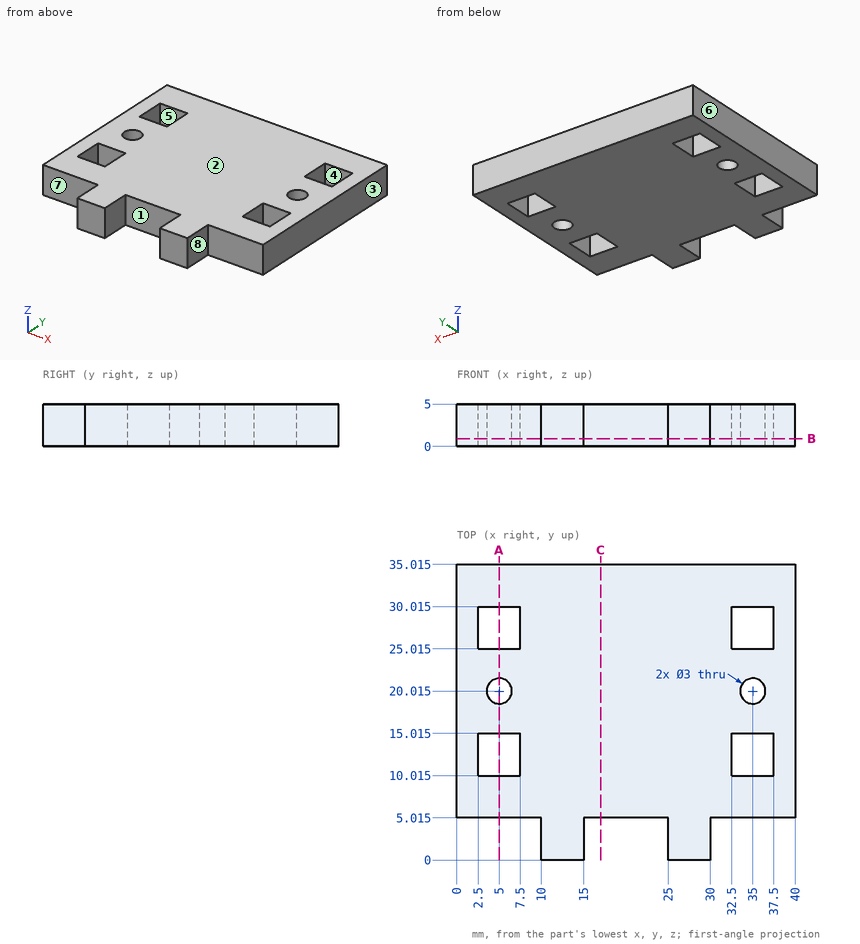
Part print with two shaded views. Sizes in mm from the minimum x, y, z corner. A direction names the side the tool comes from. Round coordinates to 2 decimals unless told otherwise and drop trailing zeros. Order: outer loops, then holes, each group sorted by start corner. A loop starts at its lowest first (then second) coordinate and runs counter-clockwise, first axis right, second up. Notation, with made-up numbers: M 62.5,62.25 L 112.5,62.25 A7 cw 112.5,71.25 Z; hole C -19,31 d9. An arc over 180 degrees is marked long. Use CSV: the item, a comma, the result in double quotes. Start each with the question number.
(1) Tool access for the marked faces 5, 6, 7 and 8: list every direction of +Z, -Z, +X, -X, +Y, -Y with a clear straight run to the whole face (end or side of a thin tool).
(2) Flat gauge pin, fed straight in: P1, Ø1.5, axis at x = 35, z = 3, coming from the -Y side (1 decimal). Where does the tip first touch, or does it go through?
(3) Cut at A-A on x = 5. List the corners of the cut face in (y, z) (1 decimal).
(4) Cut at C-C on x = 17. List the corners of the cut face in (y, z) (1 decimal), then the cut area to 3 significant figures.
(5) Cut at B-B on z = 0.9. State how many separate pieces and enclosed holes the cut face has, then the cut area to 3 significant figures.
(6) Drill centre lines: probe 1 along Y at (x, z) = (35, 2.4) (1 decimal); probe 2 along X at (y, z) = (13, 0.5); probe 3 along X at (y, z) = (3.5, 2.6). Where is each one in solid material? Low to high.
(7) Mould opens along X. For the marked faces 1, 2, 3 and 4 say: +X half, -X half, draft (parallel to the pull), parting line (faces both ways), or undercut.
Findings:
1,face 5,"+Z, -Z"
1,face 6,"+Z, -Z, -X, +Y, -Y"
1,face 7,"+Z, -Z, -X, -Y"
1,face 8,"+Z, -Z, +X, -Y"
2,P1,"stops at y = 5"
3,outline,"M 5,0 L 10,0 L 10,5 L 5,5 Z; M 15,0 L 18.5,0 L 18.5,5 L 15,5 Z; M 21.5,0 L 25,0 L 25,5 L 21.5,5 Z; M 30,0 L 35,0 L 35,5 L 30,5 Z"
4,outline,"M 5,0 L 35,0 L 35,5 L 5,5 Z"
4,area,"150 mm^2"
5,separate pieces,"1"
5,enclosed holes,"6"
5,area,"1,140 mm^2"
6,probe 1,"y = 5 to 10, 15 to 18.5, 21.5 to 25, 30 to 35"
6,probe 2,"x = 0 to 2.5, 7.5 to 32.5, 37.5 to 40"
6,probe 3,"x = 10 to 15, 25 to 30"
7,face 1,"undercut"
7,face 2,"draft"
7,face 3,"+X half"
7,face 4,"undercut"
